The drawing under review shows one solid part. Ordinate dimensions are in mm from its lowest x, y, z. A direction names the side the tool comes from. Coordinates: 2 decimals unless noted, no trailing zeros. Write each loop counter-clockwise with the first axis right and the second up, starting at its lowest first coordinate (ties: lowest second). Pieces come first, ordered by that corner, then holes. Notation, with made-up numbers: (48.5, -2) - (61.5, -2) arc R11 ccw to (61.5, 7) - close; hole circle Ø7 at (-27.75, 37.25). An arc over 180 degrees is marked (long way). Answer as CSV lines item,"result". Start each with the question number.
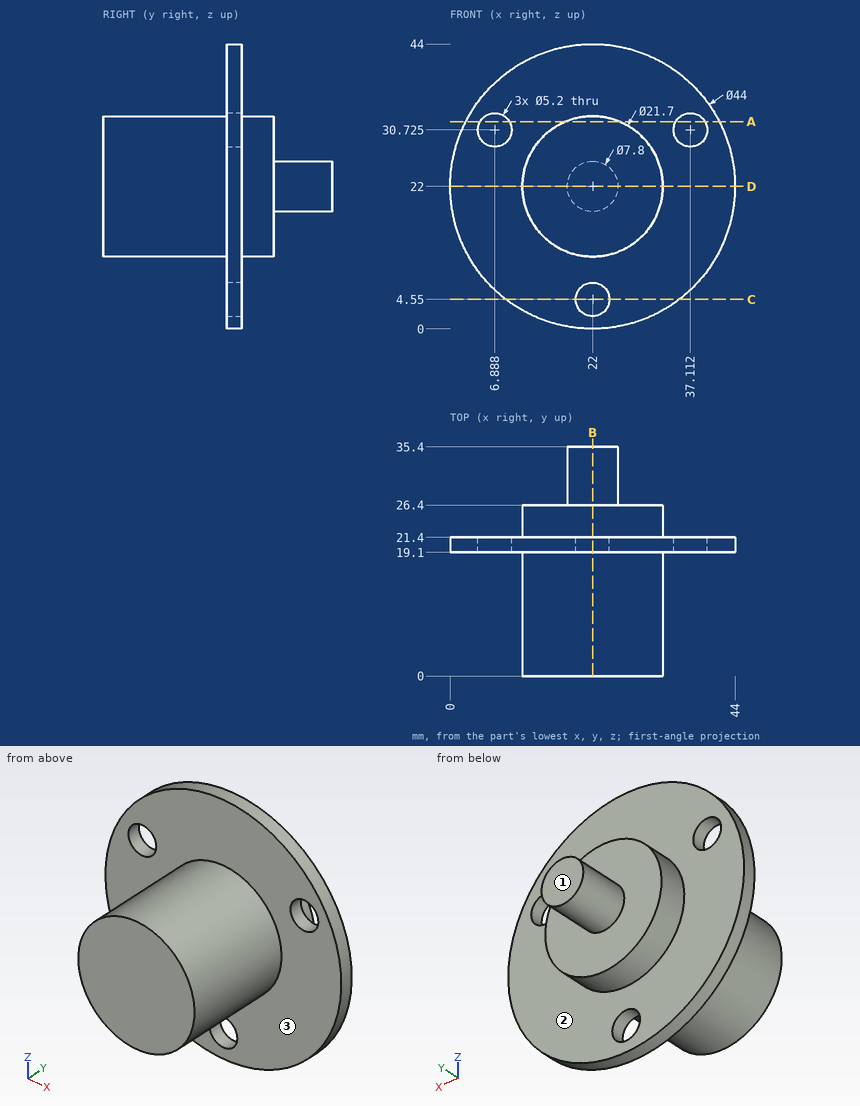
(1) Add section A-A on z = 32. Give the boundary of the cut face in (x, y).
(2) For the marked faces 1, 2 and 3, list the 3-axis set-ups (+Z, -Z, +X, -X, +Y, -Y) from which the entire face can be reached by the end or side of a thin tool; tool diameter is ignored.
(3) Add section D-D on z = 22. Give the boundary of the cut face in (x, y).
(4) Add section B-B on x = 22. Give the boundary of the cut face in (y, z), then the cut area to 3 significant figures.
(5) For pin 1 (10 mm diameter, centred on x = 26.5, z = 8.5, fed in from -Y); pin 2 (7 mm diameter, centred on x = 6.89, z = 30.72, fed in from -Y); pin 3 (3 mm diameter, centred on y = 25, z = 8.5, fed in from +X); pin 4 (5 mm diameter, centred on y = 6.5, z = 31.5, fed in from -X), all flat-tipped, find the tip position at first contact; note any pin that passes through.
(6) Add section C-C on z = 4.55. Give the boundary of the cut face in (x, y).
(7) Wall thickness on line 1 (Y direction, x = 27, z = 35); line 2 (Z direction, x = 21.5, y = 2); line 3 (X direction, y = 20.6, z = 4.55): over which ranges is each line inside the solid? List them lowest first.
Reported:
1,outline,"(2.4, 19.1) - (4.62, 19.1) - (4.62, 21.4) - (2.4, 21.4) - close; (9.15, 19.1) - (17.79, 19.1) - (17.79, 0) - (26.21, 0) - (26.21, 19.1) - (34.85, 19.1) - (34.85, 21.4) - (26.21, 21.4) - (26.21, 26.4) - (17.79, 26.4) - (17.79, 21.4) - (9.15, 21.4) - close; (39.38, 19.1) - (41.6, 19.1) - (41.6, 21.4) - (39.38, 21.4) - close"
2,face 1,"+Z, -Z, +X, -X, +Y"
2,face 2,"+Y"
2,face 3,"-Y"
3,outline,"(0, 19.1) - (11.15, 19.1) - (11.15, 0) - (32.85, 0) - (32.85, 19.1) - (44, 19.1) - (44, 21.4) - (32.85, 21.4) - (32.85, 26.4) - (25.9, 26.4) - (25.9, 35.4) - (18.1, 35.4) - (18.1, 26.4) - (11.15, 26.4) - (11.15, 21.4) - (0, 21.4) - close"
4,outline,"(0, 11.15) - (19.1, 11.15) - (19.1, 7.15) - (21.4, 7.15) - (21.4, 11.15) - (26.4, 11.15) - (26.4, 18.1) - (35.4, 18.1) - (35.4, 25.9) - (26.4, 25.9) - (26.4, 32.85) - (21.4, 32.85) - (21.4, 44) - (19.1, 44) - (19.1, 32.85) - (0, 32.85) - close; (19.1, 0) - (21.4, 0) - (21.4, 1.95) - (19.1, 1.95) - close"
4,area,"682 mm²"
5,pin 1,"y = 0"
5,pin 2,"y = 19.1"
5,pin 3,"through"
5,pin 4,"x = 13.71"
6,outline,"(8.6, 19.1) - (19.4, 19.1) - (19.4, 21.4) - (8.6, 21.4) - close; (24.6, 19.1) - (35.4, 19.1) - (35.4, 21.4) - (24.6, 21.4) - close"
7,line 1,"19.1 to 21.4"
7,line 2,"11.16 to 32.84"
7,line 3,"8.6 to 19.4, 24.6 to 35.4"
